Autodesk Inventor part; units mm, degrees
ref_plane "YZ Plane" through (0, 0, 0) normal (1, 0, 0) x (0, 1, 0)
ref_plane "XZ Plane" through (0, 0, 0) normal (0, 1, 0) x (-1, 0, 0)
ref_plane "XY Plane" through (0, 0, 0) normal (0, 0, 1) x (1, 0, 0)
sketch "Sketch1" plane through (0, 0, 0) normal (0, 1, 0) x (-1, 0, 0)
  line L0 (0, 0) -> (100, 0)
  line L1 (100, 0) -> (100, -100)
  line L2 (100, -100) -> (0, -100)
  line L3 (0, -100) -> (0, 0)
  line L4 (100, 0) -> (98, 0)
  line L5 (98, 0) -> (98, -2)
  line L6 (98, -2) -> (100, -2)
  line L7 (100, -2) -> (100, 0)
  line L8 (100, -100) -> (98, -100)
  line L9 (98, -100) -> (98, -98)
  line L10 (98, -98) -> (100, -98)
  line L11 (100, -98) -> (100, -100)
  line L12 (0, -100) -> (2, -100)
  line L13 (2, -100) -> (2, -98)
  line L14 (2, -98) -> (0, -98)
  line L15 (0, -98) -> (0, -100)
  line L16 (0, 0) -> (2, 0)
  line L17 (2, 0) -> (2, -2)
  line L18 (2, -2) -> (0, -2)
  line L19 (0, -2) -> (0, 0)
  line L20 (98, -2) -> (2, -2)
  line L21 (2, -2) -> (2, -98)
  line L22 (2, -98) -> (98, -98)
  line L23 (98, -98) -> (98, -2)
  dimension "d0" = 100
  dimension "d1" = 100
  dimension "d2" = 2
  dimension "d3" = 2
  dimension "d4" = 2
  dimension "d5" = 2
  dimension "d6" = 2
  dimension "d7" = 2
  dimension "d8" = 2
  dimension "d9" = 2
extrude "Extrusion1" add sketch "Sketch1" against normal blind 48 contours L0 L17 L18 L3 | L0 L5 L20 L17 | L18 L21 L14 L3 | L0 L1 L6 L5 | L14 L13 L2 L3 | L6 L1 L10 L23 | L22 L9 L2 L13 | L10 L1 L2 L9
sketch "Sketch2" plane through (0, -48, 0) normal (0, -1, 0) x (1, 0, 0)
  line L0 (0, 0) -> (-100, 0)
  line L1 (-100, 0) -> (-100, -100)
  line L2 (-100, -100) -> (0, -100)
  line L3 (0, -100) -> (0, 0)
extrude "Extrusion2" add sketch "Sketch2" along normal blind 2
extrude "Extrusion3" [suppressed]
sketch "Sketch4" plane through (0, 48, 0) normal (0, 1, 0) x (1, 0, 0)
  line L0 (-100, 100) -> (0, 100)
  line L1 (0, 100) -> (0, 0)
  line L2 (0, 0) -> (-100, 0)
  line L3 (-100, 0) -> (-100, 100)
extrude "Extrusion4" [suppressed]
properties part number "Box"
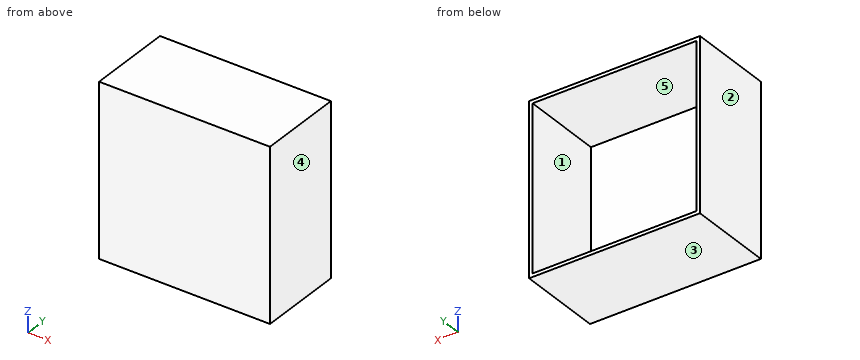
Here's how the part is built. I have some questions about the finished solid (model axes, mm). Face numbers are marked on the shaded views. A direction names the side the tool comes from. Coordinates: 2 decimals unless noted, no trailing zeros. Loops run counter-clockwise (first coordinate to the right, second up) from the corner with the lowest first, then second, coordinate; pieces in that order, holes last.
1. Imagine slicing it at A-A, the plane y = -45.5. Please give me the cut outline in (x, z).
2. Imagine slicing it at C-C, the plane x = -15. Please give me the cut outline in (y, z).
3. If we mould it in two halves opening along Z, with no side actions, what happens to the marked faces 3, 4 and 5? For each: pulls with the +Z half, pulls with the -Z half, needs draft (parallel to the pull), parting line crosses it, or undercut.
4. For the marked faces 1 and 2, which set-ups out of +Z, -Z, +X, -X, +Y, -Y let a thin tool reach every point of the face, with its end or its side?
5. Imagine slicing it at B-B, the plane z = -71. Please give me the cut outline in (x, y).
6. For P1, Ø3, axis at x = -32, z = -65.5, coming from the +Y side, with a flat end and sliding along its axis, tell me the tip position at first contact or that it passes through.
7. I need wall thicknesses on L1, parallel to X at y = -8, z = -67; L2, parallel to Y at x = -76.5, z = -87.5. Which ranges of each line are inside material? Lowest first, please.
Taken from the geometry:
1. outline: (-100, -100) - (0, -100) - (0, 0) - (-100, 0) - close; hole (-98, -98) - (-2, -98) - (-2, -2) - (-98, -2) - close
2. outline: (-50, -100) - (0, -100) - (0, -98) - (-48, -98) - (-48, -2) - (0, -2) - (0, 0) - (-50, 0) - close
3. face 3: pulls with the -Z half
3. face 4: needs draft
3. face 5: undercut
4. face 1: +Y
4. face 2: +Z, -Z, -X, +Y, -Y
5. outline: (-100, -50) - (0, -50) - (0, 0) - (-2, 0) - (-2, -48) - (-98, -48) - (-98, 0) - (-100, 0) - close
6. P1: stops at y = -48
7. L1: x = -100 to -98, -2 to 0
7. L2: y = -50 to -48
